Autodesk Inventor part; units mm, degrees
ref_plane "YZ Plane" through (0, 0, 0) normal (1, 0, 0) x (0, 1, 0)
ref_plane "XZ Plane" through (0, 0, 0) normal (0, 1, 0) x (-1, 0, 0)
ref_plane "XY Plane" through (0, 0, 0) normal (0, 0, 1) x (1, 0, 0)
sketch "Sketch1" plane through (0, 0, 0) normal (0, 1, 0) x (-1, 0, 0)
  line L0 (50.8, 53.975) -> (-50.8, 53.975)
  line L1 (-50.8, 53.975) -> (-50.8, -53.975)
  line L2 (-50.8, -53.975) -> (50.8, -53.975)
  line L3 (50.8, -53.975) -> (50.8, 53.975)
  point P0 (0, 0)
  dimension "d0" = 107.95
  dimension "d1" = 101.6
  dimension "d2" = 50.8
  dimension "d3" = 53.975
extrude "Extrusion1" add sketch "Sketch1" along normal blind 3.175
sketch "Sketch4" plane through (0, 3.175, 0) normal (0, 1, 0) x (1, 0, 0)
  circle A0 centre (44.45, 47.625) radius 3.175
  circle A1 centre (44.45, -47.625) radius 3.175
  circle A2 centre (-41.91, -29.845) radius 3.175
  line L0 (50.8, 53.975) -> (-50.8, 53.975)
  line L1 (50.8, -53.975) -> (50.8, 53.975)
  line L2 (-50.8, -53.975) -> (50.8, -53.975)
  line L3 (-50.8, 53.975) -> (-50.8, -53.975)
  circle A3 centre (-41.91, 29.845) radius 3.175
  point P0 (0, 0)
  dimension "d20" = 6.35
  dimension "d21" = 6.35
  dimension "d22" = 6.35
  dimension "d23" = 6.35
  dimension "d24" = 6.35
  dimension "d25" = 6.35
  dimension "d26" = 6.35
  dimension "d27" = 24.13
  dimension "d28" = 8.89
  dimension "d32" = 6.35
  dimension "d33" = 24.13
  dimension "d34" = 8.89
extrude "Extrusion6" [suppressed]
fillet "Fillet1" radius 3.175 4 edges at (-50.8, 1.5875, 53.975) (50.8, 1.5875, 53.975) (50.8, 1.5875, -53.975) (-50.8, 1.5875, -53.975)
sketch "Sketch6" plane through (0, 0, 0) normal (0, -1, 0) x (1, 0, 0)
  circle A0 centre (-33.4435, 47.625) radius 1.4224
  circle A1 centre (-26.7125, 40.894) radius 1.4224
  line L0 (-26.7125, -40.3479) -> (-12.425, -40.3479)
  circle A2 centre (-19.9815, 47.625) radius 1.4224
  circle A3 centre (-35.08, 10.6518) radius 1.4224
  circle A4 centre (-26.06, 10.6518) radius 1.4224
  circle A5 centre (-35.08, -17.3326) radius 1.4224
  circle A6 centre (-26.06, -17.3326) radius 1.4224
  circle A7 centre (-33.4435, -53.975) radius 1.4224
  circle A8 centre (-26.7125, -47.244) radius 1.4224
  circle A9 centre (-19.9815, -53.975) radius 1.4224
  point P0 (0, 0)
extrude "Extrusion7" cut sketch "Sketch6" against normal through all
equation "\"d21\" = d20"
equation "\"d22\" = d20"
equation "\"d24\" = d23"
equation "\"d25\" = d24"
equation "\"d26\" = d23"
equation "\"d32\" = d20"
equation "\"d33\" = d27"
equation "\"d34\" = d28"
properties part number "Base plate" material "Aluminum 6061"
For this review, take the finished solid that the model builds, in its own axes (mm). Round coordinates to 2 decimals unless told otherwise and drop trailing zeros. Answer as CSV lines item,"result". Start each with the question number.
(1) For line 1 (Z direction, x = -35.08, y = 1.85) (3 decimals); line 2 (Z direction, x = -26.06, y = 2) (3 decimals); line 3 (X direction, y = 2.5, z = -17), list the stretches that pass through material, from the lowest coordinate up.
(2) For pin 1 (1.7 mm diameter, centred on x = -26.71, z = -47.24, fed in from -Y), flat-tipped, find the tip position at first contact; note if it passes through.
(3) Mouldability with a two-part tool opening along X and no side actions: class faces 1 (the cylindrical face through (-21.4, 1.6, 47.7)), 2 (the cylindrical face through (-49.845, 1.61, -53.07)), 3 (the cylindrical face through (-36.128, 1.565, -16.371)), 4 (the flat face through (-27, 2, -53.975)) as +X half, -X half, draft (parallel to the pull), parting line (faces both ways), or undercut.
From the geometry:
1,line 1,"z = -53.975 to -18.755, -15.91 to 9.229, 12.074 to 53.975"
1,line 2,"z = -53.975 to -48.508, -45.98 to -18.755, -15.91 to 9.229, 12.074 to 39.63, 42.158 to 53.975"
1,line 3,"x = -50.8 to -36.46, -33.7 to -27.44, -24.68 to 50.8"
2,pin 1,"passes through"
3,face 1,"undercut"
3,face 2,"-X half"
3,face 3,"undercut"
3,face 4,"draft"
